Design review of the part built by this model. Coordinates are the model's own, in mm. A direction names the side the tool comes from. Round coordinates to 2 decimals unless told otherwise and drop trailing zeros. Loops run counter-clockwise (first coordinate to the right, second up) from the corner with the lowest first, then second, coordinate; pieces in that order, holes last. Notation, with made-up numbers: (-9.5, -14.5) - (8.5, -14.5) arc R22 ccw to (8.5, 0.5) - close; hole circle Ø11 at (30.25, -12.5). An arc over 180 degrees is marked (long way). Answer as CSV lines item,"result". Start each with the question number.
(1) Consider section A-A (x = 0). Give the boundary of the cut face in (y, z).
(2) For faces 5 (the flat face through (-10, -13, 18)), 6 (the flat face through (2, 20, 8)), 7 (the flat face through (-10, 15, 8)), 8 (the cylindrical face through (-1.27, 0.97, 5.08)), list the 3-axis set-ups (+Z, -Z, +X, -X, +Y, -Y) from which the entire face can be reached by the end or side of a thin tool; tool diameter is ignored.
(3) Consider section B-B (y = -10). Give the boundary of the cut face in (x, z).
(4) Consider section C-C (z = 12). Count the separate pieces of the cut face and the enclosed holes in it, and give its area (3 significant figures).
(5) Consider section D-D (y = 11.5). Give the boundary of the cut face in (x, z) (3 decimals), and give its area (3 significant figures).
(6) Mouldability with a two-part tool opening along Y and no side actions: class faces 1 (the flat face through (-10, -15, 8)), 2 (the flat face through (18.3, -5, 15.6)), 3 (the cylindrical face through (8.65, 15.32, 12.92)), 4 (the flat face through (-2, 20, 8)) as released by +Y, released by -Y, zero draft, split by the parting line, or undercut.
(7) For P1, Ø12, axis at y = 15.5, z = 3, coming from the -X side; P2, Ø4, axis at x = -10.5, z = 5, coming from the +Y side; P3, Ø5, axis at y = -8, z = 14, coming from the +X side, all flat-tipped, find the tip position at first contact; note any pin that passes through.
(8) Wall thickness on L1, parallel to Y at x = 0, z = 3; L2, parallel to X at y = -15, z = 14; L3, parallel to Y at x = -10.25, z = 14.75: over which ranges is each line inside the solid? List them lowest first.
from build123d import *

# Parameters (mm, degrees)
SKETCH_R        = 22
PAD_DEPTH       = 15
PAD001_DEPTH    = 15
POCKET_DEPTH    = 30.001
SKETCH003_R     = 2.5
PAD002_DEPTH    = 3
SKETCH004_R     = 1.6
POCKET001_DEPTH = 10
POCKET002_DEPTH = 15.001
SKETCH006_W     = 16
SKETCH006_H     = 6.5
POCKET003_DEPTH = 12
PAD003_DEPTH    = 1.5
PAD004_DEPTH    = 10
SKETCH009_R     = 1.6
POCKET004_DEPTH = 16.4648979005
SKETCH010_R     = 1.6
POCKET005_DEPTH = 10
CHAMFER_SIZE    = 0.3
CHAMFER001_SIZE = 0.3
CHAMFER002_SIZE = 0.3
CHAMFER003_SIZE = 0.3
CHAMFER004_SIZE = 0.3
CHAMFER005_SIZE = 0.3


with BuildPart() as part:
    # Sketch → Pad (new body)
    with BuildSketch(Plane.XY):
        Circle(SKETCH_R)
    extrude(amount=PAD_DEPTH)

    # Sketch001 → Pad001 (new body)
    with BuildSketch(Plane.XY.offset(15)):
        with BuildLine():
            ThreePointArc((-15.0996688705, 16), (-22, 0), (-15.0996688705, -16))
            Line((-15.0996688705, 16), (-15.0996688705, -16))
        make_face()
    extrude(amount=PAD001_DEPTH)

    # Sketch002 → Pocket (cut, through all)
    with BuildSketch(Plane.XY.offset(30)):
        with BuildLine():
            ThreePointArc((-20.4939015319, 8), (-22, 0), (-20.4939015319, -8))
            Line((-20.4939015319, -8), (-17.0996688705, -8))
            Line((-17.0996688705, 8), (-17.0996688705, -8))
            Line((-20.4939015319, 8), (-17.0996688705, 8))
        make_face()
    extrude(amount=-POCKET_DEPTH, mode=Mode.SUBTRACT)

    # Sketch003 → Pad002 (new body)
    with BuildSketch(Plane.XY.offset(15)):
        with Locations((-10.25, 15.25)):
            Circle(SKETCH003_R)
        with Locations((10.25, 15.25)):
            Circle(SKETCH003_R)
        with Locations((-10.25, -15.25)):
            Circle(SKETCH003_R)
        with Locations((10.25, -15.25)):
            Circle(SKETCH003_R)
    extrude(amount=PAD002_DEPTH)

    # Sketch004 → Pocket001 (cut)
    with BuildSketch(Plane.XY.offset(18)):
        with Locations((-10.25, 15.25)):
            Circle(SKETCH004_R)
        with Locations((10.25, 15.25)):
            Circle(SKETCH004_R)
        with Locations((-10.25, -15.25)):
            Circle(SKETCH004_R)
        with Locations((10.25, -15.25)):
            Circle(SKETCH004_R)
    extrude(amount=-POCKET001_DEPTH, mode=Mode.SUBTRACT)

    # Sketch005 → Pocket002 (cut, through all)
    with BuildSketch(Plane.XY.offset(15)):
        with BuildLine():
            ThreePointArc((2, 21.9089023002), (0, 22), (-2, 21.9089023002))
            Line((-2, 21.9089023002), (-2, 17.9089023002))
            Line((-2, 17.9089023002), (2, 17.9089023002))
            Line((2, 21.9089023002), (2, 17.9089023002))
        make_face()
    extrude(amount=-POCKET002_DEPTH, mode=Mode.SUBTRACT)

    # Sketch006 → Pocket003 (cut)
    with BuildSketch(Plane(origin=(-17.0996688705, 0, 0), x_dir=(0, -1, 0), z_dir=(-1, 0, 0))):
        with Locations((0, 3.25)):
            Rectangle(SKETCH006_W, SKETCH006_H)
    extrude(amount=-POCKET003_DEPTH, mode=Mode.SUBTRACT)

    # Sketch007 → Pad003 (new body)
    with BuildSketch(Plane.XY.offset(15)):
        with BuildLine():
            ThreePointArc((21.4242852856, -5), (22, 0), (21.4242852856, 5))
            Line((21.4242852856, 5), (20.4242852856, 5))
            Line((20.4242852856, 5), (20.4242852856, -5))
            Line((20.4242852856, -5), (21.4242852856, -5))
        make_face()
    extrude(amount=PAD003_DEPTH)

    # Sketch008 → Pad004 (new body)
    with BuildSketch(Plane.XZ.offset(5)):
        Polygon((20.4242852856, 16.5), (13.4242852856, 15), (20.4242852856, 15), align=None)
    extrude(amount=-PAD004_DEPTH)

    # Sketch009 → Pocket004 (cut, through all)
    with BuildSketch(Plane(origin=(-2.4838118655, 0, 11.591122039), x_dir=(0.9778024141, 0, 0.2095290887), z_dir=(-0.2095290887, 0, 0.9778024141))):
        with Locations((21.4281454222, 0)):
            Circle(SKETCH009_R)
    extrude(amount=-POCKET004_DEPTH, mode=Mode.SUBTRACT)

    # Sketch010 → Pocket005 (cut)
    with BuildSketch(Plane(origin=(0, 0, 0), x_dir=(1, 0, 0), z_dir=(0, 0, -1))):
        Circle(SKETCH010_R)
    extrude(amount=-POCKET005_DEPTH, mode=Mode.SUBTRACT)

    # Chamfer
    chamfer_edges = [part.edges().sort_by_distance(p)[0] for p in [
        (8.65, 15.25, 18),
    ]]
    chamfer(chamfer_edges, length=CHAMFER_SIZE)

    # Chamfer001
    chamfer001_edges = [part.edges().sort_by_distance(p)[0] for p in [
        (-11.85, 15.25, 18),
    ]]
    chamfer(chamfer001_edges, length=CHAMFER001_SIZE)

    # Chamfer002
    chamfer002_edges = [part.edges().sort_by_distance(p)[0] for p in [
        (-11.85, -15.25, 18),
    ]]
    chamfer(chamfer002_edges, length=CHAMFER002_SIZE)

    # Chamfer003
    chamfer003_edges = [part.edges().sort_by_distance(p)[0] for p in [
        (8.65, -15.25, 18),
    ]]
    chamfer(chamfer003_edges, length=CHAMFER003_SIZE)

    # Chamfer004
    chamfer004_edges = [part.edges().sort_by_distance(p)[0] for p in [
        (16.904197, 0, 15.745695),
    ]]
    chamfer(chamfer004_edges, length=CHAMFER004_SIZE)

    # Chamfer005
    chamfer005_edges = [part.edges().sort_by_distance(p)[0] for p in [
        (-1.6, 0, 0),
    ]]
    chamfer(chamfer005_edges, length=CHAMFER005_SIZE)


solid = part.part
Determined:
1,outline,"(-22, 0) - (-1.9, 0) - (-1.6, 0.3) - (-1.6, 10) - (1.6, 10) - (1.6, 0.3) - (1.9, 0) - (17.91, 0) - (17.91, 15) - (-22, 15) - close"
2,face 5,"+Z, +X, +Y, -Y"
2,face 6,"+Z, -Z, +Y"
2,face 7,"+Z"
2,face 8,"-Z"
3,outline,"(-19.6, 0) - (19.6, 0) - (19.6, 15) - (-15.1, 15) - (-15.1, 30) - (-19.6, 30) - close"
4,separate pieces,"1"
4,enclosed holes,"5"
4,area,"1,390 mm^2"
5,outline,"(-18.755, 0) - (18.755, 0) - (18.755, 15) - (-15.1, 15) - (-15.1, 30) - (-18.755, 30) - close"
5,area,"617 mm^2"
6,face 1,"undercut"
6,face 2,"released by -Y"
6,face 3,"undercut"
6,face 4,"zero draft"
7,P1,"stops at x = -19.84"
7,P2,"stops at y = 20.29"
7,P3,"stops at x = 21.3"
8,L1,"y = -22 to -1.6, 1.6 to 17.91"
8,L2,"x = -16.09 to -11.83, -8.67 to 8.67, 11.83 to 16.09"
8,L3,"y = -19.47 to -16.85, -13.65 to 13.65, 16.85 to 19.47"
